Read the model definition and answer for the solid it produces. Units are mm, in the model's axes. A direction names the side the tool comes from. Give positions to 0.01 mm unless a question says otherwise; leave off trailing zeros. Loops run counter-clockwise (first coordinate to the right, second up) from the corner with the lowest first, then second, coordinate; pieces in that order, holes last. Notation, with made-up numbers: (-33, 56.25) - (-12, 56.25) arc R9 ccw to (-12, 60.25) - close; hole circle Ø5 at (60, -7.5). An arc over 180 degrees is marked (long way). Use a Markdown table: item, result. Add a question column.
Item 1: Each of these flat-tipped pins is pushed along its axis until it touches: P1, Ø2, axis at x = 10, z = 0, coming from the -Y side; P2, Ø0.6, axis at x = 4, z = -2, coming from the +Y side; P3, Ø2, axis at x = 9.5, z = -4.5, coming from the +Y side; P4, Ø9, axis at y = -8, z = -7.5, coming from the +X side. Where does it stop, or does it pass through?
Item 2: A cutting plane is placed at B-B (x = 10). Determine the outline of the cut face in (y, z).
Item 3: A cutting plane is placed at D-D (z = -6.75). Determine the outline of the cut face in (x, y).
Item 4: Which of the six approach directions +Z, -Z, +X, -X, +Y, -Y give full straight-line access (tool end or side, diameter ignored) to faces 1 (the face through (2, 40, 10)), 2 (the face through (8, -45.5, 0)), 3 (the face through (4, 37, 0))?
Item 5: Consider probe 1 along Y at (x, z) = (2.5, 11.7); probe 2 along Y at (x, z) = (2.5, -8.25); probe 3 along X at (y, z) = (20.5, -9.5). Determine where each line is inside the solid, lowest interval first. Write a range as [from, to].
Item 6: A cutting plane is placed at C-C (y = 44.5). Determine the outline of the cut face in (x, z), plus the area to 3 significant figures.
Item 7: A cutting plane is placed at A-A (z = 0). Determine the outline of the cut face in (x, y), plus the area to 3 significant figures.
Item 8: For a pull along Y with two mould halves and no side action, classify faces 4 (the face through (2, 47.5, -12)), 5 (the face through (3, -4, 15)), 6 (the face through (7, -47.5, 0)), 7 (the face through (2.37, -44.01, 0.21)) as +Y half, -Y half, draft (parallel to the pull), parting line (faces both ways), or undercut.
from build123d import *

# Parameters (mm, degrees)
SKETCH2_W                       = 30
SKETCH2_H                       = 95
BOSS_EXTRUDE1_DEPTH             = 5
F_2MM_DIAMETER_HOLE_D           = 2
SKETCH6_W                       = 30
SKETCH6_H                       = 2
BOSS_EXTRUDE2_DEPTH             = 10
F_3_32_0_09375_DIAMETER_HOLE2_D = 2.38125
SKETCH10_W                      = 20
SKETCH10_H                      = 15
CUT_EXTRUDE3_DEPTH              = 3
SKETCH11_W                      = 20
SKETCH11_H                      = 10.5
CUT_EXTRUDE4_DEPTH              = 52.237193522
F_2MM_DIAMETER_HOLE2_D          = 2


with BuildPart() as part:
    # Sketch2 → Boss-Extrude1 (new body)
    with BuildSketch(Plane(origin=(0, 0, 0), x_dir=(0, 0, -1), z_dir=(1, 0, 0))):
        Rectangle(SKETCH2_W, SKETCH2_H)
    extrude(amount=BOSS_EXTRUDE1_DEPTH)

    # 2mm Diameter Hole (through all)
    with Locations(Plane(origin=(0, 0, -15), x_dir=(-1, 0, 0), z_dir=(0, 0, -1))):
        with Locations((-2.5, 44.5)):
            Hole(F_2MM_DIAMETER_HOLE_D / 2)

    # Sketch6 → Boss-Extrude2 (add)
    with BuildSketch(Plane(origin=(5, 0, 0), x_dir=(0, 0, -1), z_dir=(1, 0, 0))):
        with Locations((0, -46.5)):
            Rectangle(SKETCH6_W, SKETCH6_H)
    extrude(amount=BOSS_EXTRUDE2_DEPTH)

    # 3/32 (0.09375) Diameter Hole2 (through all)
    with Locations(Plane(origin=(0, -45.5, 0), x_dir=(1, 0, 0), z_dir=(0, 1, 0))):
        with Locations((10, 0)):
            Hole(F_3_32_0_09375_DIAMETER_HOLE2_D / 2)

    # Sketch10 → Cut-Extrude3 (cut)
    with BuildSketch(Plane.ZY):
        with Locations((0, 40)):
            Rectangle(SKETCH10_W, SKETCH10_H)
    extrude(amount=-CUT_EXTRUDE3_DEPTH, mode=Mode.SUBTRACT)

    # Sketch11 → Cut-Extrude4 (cut, through all)
    with BuildSketch(Plane.ZY.offset(-3)):
        with Locations((0, 42.25)):
            Rectangle(SKETCH11_W, SKETCH11_H)
    extrude(amount=-CUT_EXTRUDE4_DEPTH, mode=Mode.SUBTRACT)

    # 2mm Diameter Hole2 (through all)
    with Locations(Plane(origin=(0, 0, -15), x_dir=(-1, 0, 0), z_dir=(0, 0, -1))):
        with Locations((-2.5, -45)):
            Hole(F_2MM_DIAMETER_HOLE2_D / 2)


solid = part.part
Geometry says:
| question | item | result |
|---|---|---|
| 1 | P1 | through |
| 1 | P2 | y = 37 |
| 1 | P3 | y = -45.5 |
| 1 | P4 | x = 5 |
| 2 | outline | (-47.5, -15) - (-45.5, -15) - (-45.5, -1.19) - (-47.5, -1.19) - close; (-47.5, 1.19) - (-45.5, 1.19) - (-45.5, 15) - (-47.5, 15) - close |
| 3 | outline | (0, -47.5) - (15, -47.5) - (15, -45.5) - (5, -45.5) - (5, 37) - (3, 37) - (3, 32.5) - (0, 32.5) - close; hole circle Ø2 at (2.5, -45) |
| 4 | face 1 | -X, +Y |
| 4 | face 2 | +Z, -Z, +X, +Y |
| 4 | face 3 | +X, -X, +Y |
| 5 | probe 1 | [-47.5, -46], [-44, 43.5], [45.5, 47.5] |
| 5 | probe 2 | [-47.5, -46], [-44, 32.5] |
| 5 | probe 3 | [0, 5] |
| 6 | outline | (0, -15) - (1.5, -15) - (1.5, -10) - (0, -10) - close; (0, 10) - (1.5, 10) - (1.5, 15) - (0, 15) - close; (3.5, -15) - (5, -15) - (5, -10) - (3.5, -10) - close; (3.5, 10) - (5, 10) - (5, 15) - (3.5, 15) - close |
| 6 | area | 30.0 mm² |
| 7 | outline | (0, -47.5) - (8.81, -47.5) - (8.81, -45.5) - (5, -45.5) - (5, 37) - (3, 37) - (3, 32.5) - (0, 32.5) - close; (11.19, -47.5) - (15, -47.5) - (15, -45.5) - (11.19, -45.5) - close; hole circle Ø2 at (2.5, -45) |
| 7 | area | 421 mm² |
| 8 | face 4 | +Y half |
| 8 | face 5 | draft |
| 8 | face 6 | -Y half |
| 8 | face 7 | undercut |
